from build123d import *

# Parameters (mm, degrees)
F0_W     = 368.7085997245
F0_H     = 208.0708047671
F0_W_2   = 338.2285997245
F0_H_2   = 177.5908047671
F1_DEPTH = 185.42
F3_W     = 152.4
F3_H     = 14.9174671465
F4_DEPTH = 88.9
F5_DEPTH = 14.224
F6_DEPTH = 25.4
F7_DEPTH = 25.4
F8_R     = 21.4933910587
F9_DEPTH = 469.9


with BuildPart() as f1:
    # F0 (on Top) → F1 (new body)
    with BuildSketch(Plane.XY):
        with Locations((2.6404061785, 0.0097863376)):
            Rectangle(F0_W, F0_H)
        with Locations((2.6404061785, 0.0097863376)):
            Rectangle(F0_W_2, F0_H_2, mode=Mode.SUBTRACT)
    extrude(amount=F1_DEPTH)

    # F3 (on face) → F4 (cut)
    with BuildSketch(Plane.XY):
        with Locations((0.3421455622, -96.07069315)):
            Rectangle(F3_W, F3_H)
        Polygon((-76.1339217424, 104.031085968), (-76.1339217424, 89.1409292817), (76.6604244709, 88.854573667), (76.6604244709, 104.031085968), align=None)
    extrude(amount=F4_DEPTH, mode=Mode.SUBTRACT)

    # F5 (cut): a face of the model
    f5_faces = [f1.faces().sort_by_distance(p)[0] for p in [
        (0.3421455622, -103.5294267233, 44.45),
    ]]
    extrude(f5_faces, amount=-F5_DEPTH, mode=Mode.SUBTRACT)

    # F6 (cut): a face of the model
    f6_faces = [f1.faces().sort_by_distance(p)[0] for p in [
        (0.2632513642, 88.9977514744, 44.45),
    ]]
    extrude(f6_faces, amount=-F6_DEPTH, mode=Mode.SUBTRACT)

    # F7 (cut): a face of the model
    f7_faces = [f1.faces().sort_by_distance(p)[0] for p in [
        (0.2632513642, 104.031085968, 44.45),
    ]]
    extrude(f7_faces, amount=-F7_DEPTH, mode=Mode.SUBTRACT)

    # F8 (on face) → F9 (cut)
    with BuildSketch(Plane(origin=(-181.7138936837, 0, 0), x_dir=(0, -1, 0), z_dir=(-1, 0, 0))):
        with Locations((0, 92.71)):
            Circle(F8_R)
    extrude(amount=-F9_DEPTH, mode=Mode.SUBTRACT)


solid = f1.part
For this review, take the finished solid that the model builds, in its own axes (mm). A direction names the side the tool comes from. Round coordinates to 2 decimals unless told otherwise and drop trailing zeros. Write each loop counter-clockwise with the first axis right and the second up, starting at its lowest first coordinate (ties: lowest second). Pieces come first, ordered by that corner, then holes. Notation, with made-up numbers: (-3.75, -13.75) - (45.25, -13.75) arc R18 ccw to (45.25, -1.75) - close; hole circle Ø7 at (41.5, -26.75). An arc over 180 degrees is marked (long way). Write item = value, one per line. Start each with the question number.
1. Consider section D-D on z = 77. State the section outline as (x, y) points, plus the area to 3 significant figures.
2. Consider section B-B on y = 0. State the section outline as (x, z) points, plus the area to 3 significant figures.
3. For pin 1 Ø12 at (x, y) = (22.5, 97) entering from -Z, flat-tipped, find the tip position at first contact; note if it passes through.
4. Consider section A-A on z = 56.5. State the section outline as (x, y) points.
5. Draft analysis for pull direction Y (two halves, no side actions). For faces 4 (the face through (-174.201, 21.473, 93.655)), 5 (the face through (-168, -7, 0)), 6 (the face through (0, -104.026, 91)), state which applies: released by +Y, released by -Y, zero draft, split by the parting line, or undercut.
6. Consider section C-C on y = 47. State the section outline as (x, z) points.
7. For faces 1 (the face through (-1, -96, 88.9)), 2 (the face through (-12, -92, 185.42)), 3 (the face through (-166.474, -1, 71)), list the 3-axis set-ups (+Z, -Z, +X, -X, +Y, -Y) from which the entire face can be reached by the end or side of a thin tool; tool diameter is ignored.
8. Wall thickness on L1, parallel to Y at x = 152, z = 114.5; L2, parallel to X at y = -21, z = 41.5; L3, parallel to Z at x = 183.5, y = 0: over which ranges is each line inside the solid? List them lowest first.
Evaluation:
q1.outline = (-181.71, -104.03) - (-75.86, -104.03) - (-75.86, -88.79) - (-166.47, -88.79) - (-166.47, -14.67) - (-181.71, -14.67) - close; (-181.71, 14.67) - (-166.47, 14.67) - (-166.47, 88.81) - (-76.13, 88.81) - (-76.13, 89.14) - (-76.13, 104.05) - (-181.71, 104.05) - close; (76.54, -104.03) - (186.99, -104.03) - (186.99, -14.67) - (171.75, -14.67) - (171.75, -88.79) - (76.54, -88.79) - close; (76.66, 88.81) - (171.75, 88.81) - (171.75, 14.67) - (186.99, 14.67) - (186.99, 104.05) - (76.66, 104.05) - (76.66, 88.85) - close
q1.area = 11,100 mm2
q2.outline = (-181.71, 0) - (-166.47, 0) - (-166.47, 71.22) - (-181.71, 71.22) - close; (-181.71, 114.2) - (-166.47, 114.2) - (-166.47, 185.42) - (-181.71, 185.42) - close; (171.75, 0) - (186.99, 0) - (186.99, 71.22) - (171.75, 71.22) - close; (171.75, 114.2) - (186.99, 114.2) - (186.99, 185.42) - (171.75, 185.42) - close
q2.area = 4,340 mm2
q3.pin_1 = 88.9
q4.outline = (-181.71, -104.03) - (-75.86, -104.03) - (-75.86, -88.79) - (-166.47, -88.79) - (-166.47, 88.81) - (-76.13, 88.81) - (-76.13, 89.14) - (-76.13, 104.05) - (-181.71, 104.05) - close; (76.54, -104.03) - (186.99, -104.03) - (186.99, 104.05) - (76.66, 104.05) - (76.66, 88.85) - (76.66, 88.81) - (171.75, 88.81) - (171.75, -88.79) - (76.54, -88.79) - close
q5.face_4 = undercut
q5.face_5 = zero draft
q5.face_6 = released by -Y
q6.outline = (-181.71, 0) - (-166.47, 0) - (-166.47, 185.42) - (-181.71, 185.42) - close; (171.75, 0) - (186.99, 0) - (186.99, 185.42) - (171.75, 185.42) - close
q7.face_1 = -Z, +Y, -Y
q7.face_2 = +Z, +X, -X, +Y, -Y
q7.face_3 = +Z, -Z
q8.L1 = -104.03 to -88.79, 88.81 to 104.05
q8.L2 = -181.71 to -166.47, 171.75 to 186.99
q8.L3 = 0 to 71.22, 114.2 to 185.42
